from build123d import *

# Parameters (mm, degrees)
SALIENTE_EXTRUIR1_DEPTH = 25


with BuildPart() as part:
    # Croquis1 → Revolución3 (revolve)
    with BuildSketch(Plane.XY):
        Polygon((0, 0), (0, -110), (4, -106), (4, -100), (6, -100), (6, 0), align=None)
    revolve(axis=Axis((0, 0, 0), (0, -1, 0)))

    # Croquis2 → Saliente-Extruir1 (add)
    with BuildSketch(Plane(origin=(0, 0, 0), x_dir=(1, 0, 0), z_dir=(0, 1, 0))):
        Polygon((8.310422033, -5.222089521), (8.677673202, 4.585991836), (0.367251169, 9.808081357), (-8.310422033, 5.222089521), (-8.677673202, -4.585991836), (-0.367251169, -9.808081357), align=None)
    extrude(amount=SALIENTE_EXTRUIR1_DEPTH)

    # Croquis3 → Cortar-Revolución1 (revolve, cut)
    with BuildSketch(Plane(origin=(0, 0, 0), x_dir=(0, 0, -1), z_dir=(1, 0, 0))):
        Polygon((5.04976064, 27.002153948), (10.24964381, 27.002153948), (10.24964381, 24), align=None)
    revolve(axis=Axis((0, 0, 0), (0, 1, 0)), mode=Mode.SUBTRACT)


solid = part.part
Work out the finished part from the listing and answer in its coordinate system (mm). A direction names the side the tool comes from. Round coordinates to 2 decimals unless told otherwise and drop trailing zeros. Loops run counter-clockwise (first coordinate to the right, second up) from the corner with the lowest first, then second, coordinate; pieces in that order, holes last. Notation, with made-up numbers: (-32, 19.25) - (16, 19.25) arc R20 ccw to (16, 30.25) - close; hole circle Ø6 at (44, 12.5). An arc over 180 degrees is marked (long way). Use one line per item in the form item = value. Start each with the question number.
(1) Which of the six approach directions +Z, -Z, +X, -X, +Y, -Y give full straight-line access (tool end or side, diameter ignored) to faces 1 (the face through (-0.867, -102.958, -3.905)), 2 (the face through (-3.911, 12.325, -7.547))?
(2) Flat-ended cylindrical pins translate along their axes: P1, Ø10, axis at x = 2, y = -12.5, coming from the -Z side; P2, Ø5, axis at x = 4, y = -74.5, coming from the -Z side; P3, Ø6, axis at x = -6.5, z = -3, coming from the -Y side. Find the tip coordinate at first contact, or state that the pin passes through.
(3) Find section B-B on y = -16.5. Determine the outline of the cut face in (x, z).
(4) Consider line 1 (Y direction, x = -4.75, z = -2.25); line 2 (Z direction, x = 0.5, y = -81.5); line 3 (X direction, y = -102, z = -0.25). Determine where each line is inside the solid, lowest interval first.
(5) Find section A-A on y = 2. Determine the outline of the cut face in (x, z), and give its area (3 significant figures).
Answer list:
q1.face_1 = -Y
q1.face_2 = -Z, -X, +Y, -Y
q2.P1 = -6
q2.P2 = -5.81
q2.P3 = -100
q3.outline = circle Ø12 at (0, 0)
q4.line_1 = -100 to 25
q4.line_2 = -5.98 to 5.98
q4.line_3 = -3.99 to 3.99
q5.outline = (-8.68, 4.59) - (-8.31, -5.22) - (0.37, -9.81) - (8.68, -4.59) - (8.31, 5.22) - (-0.37, 9.81) - close
q5.area = 250 mm^2
